```python
from build123d import *

# Parameters (mm, degrees)
SKETCH1_R           = 2
BOSS_EXTRUDE1_DEPTH = 5
SKETCH2_W           = 116
SKETCH2_H           = 5
BOSS_EXTRUDE2_DEPTH = 35
SKETCH3_W           = 116
SKETCH3_H           = 3
SKETCH3_H_2         = 3.5
BOSS_EXTRUDE3_DEPTH = 2
FILLET1_R           = 2
FILLET2_R           = 1
FILLET3_R           = 2


with BuildPart() as part:
    # Sketch1 → Boss-Extrude1 (new body)
    with BuildSketch(Plane.XY):
        with BuildLine():
            Line((2, 0), (114, 0))
            ThreePointArc((114, 0), (115.414213562, 0.585786438), (116, 2))
            Line((116, 2), (116, 20))
            Line((116, 20), (0, 20))
            Line((0, 20), (0, 2))
            ThreePointArc((0, 2), (0.585786438, 0.585786438), (2, 0))
        make_face()
        with Locations((20, 9)):
            Circle(SKETCH1_R, mode=Mode.SUBTRACT)
        with Locations((96, 9)):
            Circle(SKETCH1_R, mode=Mode.SUBTRACT)
    extrude(amount=BOSS_EXTRUDE1_DEPTH)

    # Sketch2 → Boss-Extrude2 (add)
    with BuildSketch(Plane.XY.offset(5)):
        with Locations((58, 17.5)):
            Rectangle(SKETCH2_W, SKETCH2_H)
    extrude(amount=BOSS_EXTRUDE2_DEPTH)

    # Sketch3 → Boss-Extrude3 (add)
    with BuildSketch(Plane.XZ.offset(-15)):
        with Locations((58, 38.5)):
            Rectangle(SKETCH3_W, SKETCH3_H)
        with Locations((58, 24.25)):
            Rectangle(SKETCH3_W, SKETCH3_H_2)
    extrude(amount=BOSS_EXTRUDE3_DEPTH)

    # Fillet1
    fillet1_edges = [part.edges().sort_by_distance(p)[0] for p in [
        (0, 20, 20),
        (116, 20, 20),
        (58, 13, 40),
        (115.414213562, 0.585786438, 0),
        (58, 0, 0),
        (0.585786438, 0.585786438, 0),
        (0, 11, 0),
        (116, 11, 0),
    ]]
    fillet(fillet1_edges, radius=FILLET1_R)

    # Fillet2
    fillet2_edges = [part.edges().sort_by_distance(p)[0] for p in [
        (58, 13, 26),
        (116, 13, 24.25),
        (58, 13, 22.5),
        (0, 13, 24.25),
        (58, 13, 37),
    ]]
    fillet(fillet2_edges, radius=FILLET2_R - 0.0001)  # a hair under: the kernel refuses the full size

    # Fillet3
    fillet3_edges = [part.edges().sort_by_distance(p)[0] for p in [
        (58, 15, 5),
    ]]
    fillet(fillet3_edges, radius=FILLET3_R)


solid = part.part
```
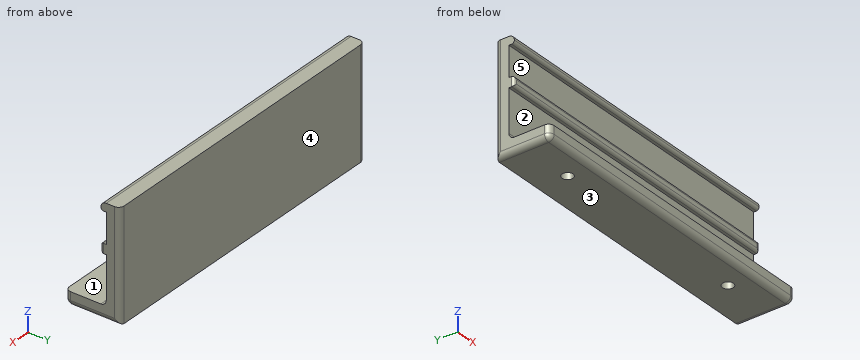
Model file for the job. Use its own axes, mm. Face numbers are marked on the shaded views. A direction names the side the tool comes from. Round coordinates to 2 decimals unless told otherwise and drop trailing zeros. Order: outer loops, then holes, each group sorted by start corner. A loop starts at its lowest first (then second) coordinate and runs counter-clockwise, first axis right, second up. Notation, with made-up numbers: (-9, -2) -> (28, -2) arc R24 cw to (28, 14) -> close; hole circle Ø5 at (-30, 45). An arc over 180 degrees is marked (long way). Use one line per item in the form item = value.
Item 1: Pull direction Z, two halves, no side cores. Call the marked faces 1, 2 and 3: released by +Z, released by -Z, zero draft, split by the parting line, or undercut.
Returned:
face_1 = released by +Z
face_2 = undercut
face_3 = released by -Z
Item 2: Cut at C-C, the plane z = 34. Write the cut outline in (x, y).
Returned:
outline = (0, 15) -> (116, 15) -> (116, 18) arc R2 ccw to (114, 20) -> (2, 20) arc R2 ccw to (0, 18) -> close
Item 3: Cut at B-B, the plane y = 9. Write the cut outline in (x, z).
Returned:
outline = (0, 2) arc R2 ccw to (2, 0) -> (18, 0) -> (18, 5) -> (0, 5) -> close; (22, 0) -> (94, 0) -> (94, 5) -> (22, 5) -> close; (98, 0) -> (114, 0) arc R2 ccw to (116, 2) -> (116, 5) -> (98, 5) -> close
Item 4: Flat gauge pins, fed straight in: pin 1 Ø8 at (x, z) = (54, 13.5) entering from -Y; pin 2 Ø9 at (x, z) = (70.5, 33.5) entering from -Y. Where does each tip first touch, or does it go through?
Returned:
pin_1 = 15
pin_2 = 13
Item 5: Drill centre lines: line 1 (Y direction, x = 20, z = 2.2); line 2 (Y direction, x = 69, z = 29); line 3 (Z direction, x = 92.5, y = 2.25). Where is each one in solid material? Low to high.
Returned:
line_1 = 0 to 7, 11 to 20
line_2 = 15 to 20
line_3 = 0 to 5
Item 6: Tool access for the marked faces 4 and 5: list every direction of +Z, -Z, +X, -X, +Y, -Y with a clear straight run to the whole face (end or side of a thin tool).
Returned:
face_4 = +Z, -Z, +X, -X, +Y
face_5 = +X, -X, -Y
